```python
from build123d import *

# Parameters (mm, degrees)
SKETCH1_R           = 2
BOSS_EXTRUDE1_DEPTH = 4


with BuildPart() as part:
    # Sketch1 → Boss-Extrude1 (new body)
    with BuildSketch(Plane.YZ):
        with BuildLine():
            Line((0, 25), (50, 25))
            ThreePointArc((50, 25), (75, 0), (50, -25))
            Line((50, -25), (0, -25))
            ThreePointArc((0, -25), (-25, 0), (0, 25))
        make_face()
        with Locations(Location((10, 19, 0), (0, 0, 270))):
            Circle(SKETCH1_R, mode=Mode.SUBTRACT)
        with Locations(Location((40, 19, 0), (0, 0, 270))):
            Circle(SKETCH1_R, mode=Mode.SUBTRACT)
        with Locations(Location((69, 0, 0), (0, 0, 270))):
            Circle(SKETCH1_R, mode=Mode.SUBTRACT)
        with Locations(Location((-19, 0, 0), (0, 0, 270))):
            Circle(SKETCH1_R, mode=Mode.SUBTRACT)
        with Locations(Location((10, -19, 0), (0, 0, 270))):
            Circle(SKETCH1_R, mode=Mode.SUBTRACT)
        with Locations(Location((40, -19, 0), (0, 0, 270))):
            Circle(SKETCH1_R, mode=Mode.SUBTRACT)
    extrude(amount=BOSS_EXTRUDE1_DEPTH)


solid = part.part
```
Can you work these out from the model? Positions are in its coordinate system, mm. Give positions to 0.01 mm unless a question says otherwise; leave off trailing zeros. Write each loop counter-clockwise with the first axis right and the second up, starting at its lowest first coordinate (ties: lowest second). Pieces come first, ordered by that corner, then holes. Notation, with made-up numbers: (80, 33.5) - (134, 33.5) arc R16 ccw to (134, 40.5) - close; hole circle Ø5 at (-28, 68.25). An arc over 180 degrees is marked (long way). Write item = value, one per line. Start each with the question number.
1. Please list where these lines run through material, in increasing order: line 1 (Y direction, x = 2.75, z = 19); line 2 (Z direction, x = 3, y = -18.5); line 3 (Z direction, x = 3, y = 70).
2. Imagine slicing it at B-B (x = 2.25). Please give me the cut outline in (y, z), and give its area (3 significant figures).
3. Imagine slicing it at D-D (y = -19). Please give me the cut outline in (x, z), and give its area (3 significant figures).
4. Imagine slicing it at C-C (z = 20). Please give me the cut outline in (x, y), and give its area (3 significant figures).
5. For pin 1 (4 mm diameter, centred on y = 7.5, z = -12, fed in from -X); pin 2 (3.5 mm diameter, centred on y = 40, z = -19, fed in from -X); pin 3 (1.5 mm diameter, centred on x = 0.5, y = -12, fed in from -Z), each with a flat end and sliding along its axis, tell me the tip position at first contact or that it passes through.
6. Thinking about a two-plate mould opening in Z: for faces 1 (the face through (1.972, -24.994, -0.55)), 2 (the face through (2, 25, -25)), 3 (the face through (2, 71, 0)), which applies, released by +Z, released by -Z, zero draft, split by the parting line, or undercut?
7. Imagine slicing it at A-A (y = 10). Please give me the cut outline in (x, z).
Worked answers:
q1.line_1 = -16.25 to 8, 12 to 38, 42 to 66.25
q1.line_2 = -16.82 to -1.94, 1.94 to 16.82
q1.line_3 = -15 to -1.73, 1.73 to 15
q2.outline = (0, -25) - (50, -25) arc R25 ccw to (50, 25) - (0, 25) arc R25 ccw to start; hole circle Ø4 at (-19, 0); hole circle Ø4 at (10, -19); hole circle Ø4 at (10, 19); hole circle Ø4 at (40, -19); hole circle Ø4 at (40, 19); hole circle Ø4 at (69, 0)
q2.area = 4,390 mm2
q3.outline = (0, -16.25) - (4, -16.25) - (4, -2) - (0, -2) - close; (0, 2) - (4, 2) - (4, 16.25) - (0, 16.25) - close
q3.area = 114 mm2
q4.outline = (0, -15) - (4, -15) - (4, 8.27) - (0, 8.27) - close; (0, 11.73) - (4, 11.73) - (4, 38.27) - (0, 38.27) - close; (0, 41.73) - (4, 41.73) - (4, 65) - (0, 65) - close
q4.area = 292 mm2
q5.pin_1 = 0
q5.pin_2 = through
q5.pin_3 = -22.33
q6.face_1 = split by the parting line
q6.face_2 = released by -Z
q6.face_3 = undercut
q7.outline = (0, -25) - (4, -25) - (4, -21) - (0, -21) - close; (0, -17) - (4, -17) - (4, 17) - (0, 17) - close; (0, 21) - (4, 21) - (4, 25) - (0, 25) - close
